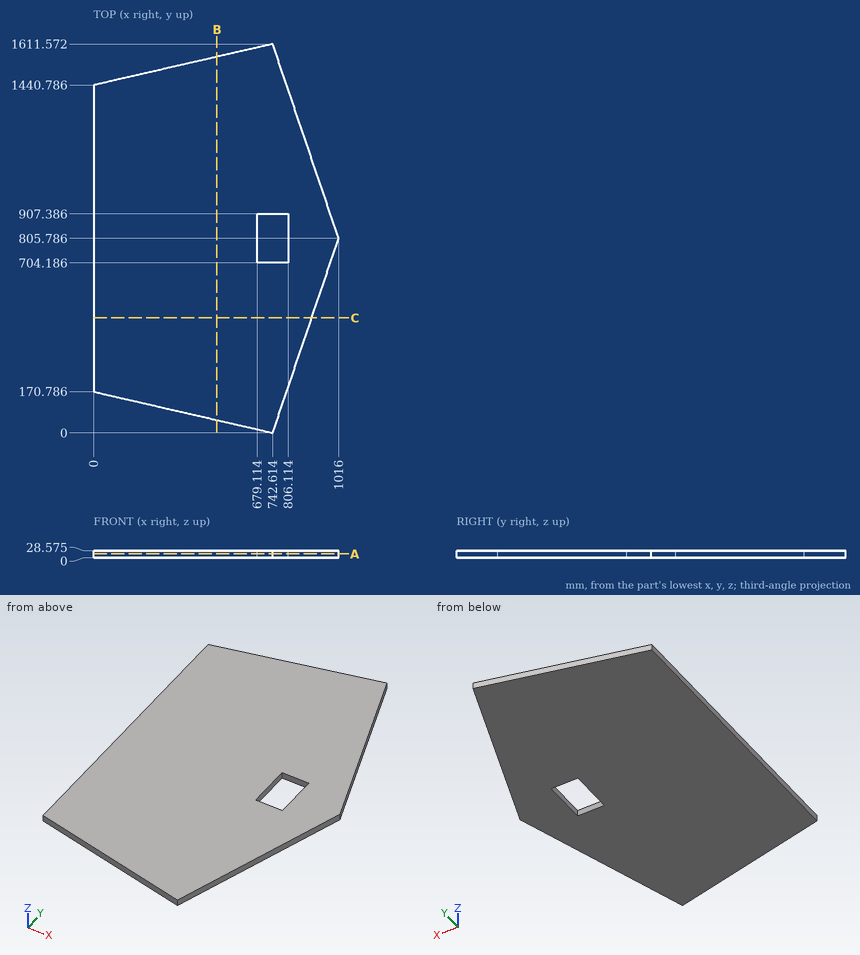
Could you check a few things on this drawing? It's one solid part, dimensions in mm from its lowest x, y, z. Coordinates: 2 decimals unless noted, no trailing zeros. Order: outer loops, then holes, each group sorted by start corner. A loop starts at its lowest first (then second) coordinate and runs counter-clockwise, first axis right, second up. Notation, with made-up numbers: M -25.75,15.25 L 22.25,15.25 A11 cw 22.25,36.25 Z; hole C -2.75,30 d4. An arc over 180 degrees is marked long. Use one line per item in the form item = value. Start each with the question number.
1. Suppose I cut it at B-B on x = 511.5. Write out the boundary of the cut face in (y, z) (1 decimal), then the cut area to 3 significant figures.
2. Suppose I cut it at C-C on y = 476.5. Write out the boundary of the cut face in (x, z) (1 decimal).
3. Suppose I cut it at A-A on z = 16.5. Write out the boundary of the cut face in (x, y) (1 decimal).
4. For pin 1 (1 mm diameter, centred on x = 492.5, z = 18.5, fed in from +Y); pin 2 (12 mm diameter, centred on x = 606, z = 16.5, fed in from -Y); pin 3 (4 mm diameter, centred on x = 250.5, z = 17.5, fed in from -Y), each with a flat end and sliding along its axis, tell me the tip position at first contact or that it passes through.
5. Please list where these lines run through material, in increasing order: line 1 (X direction, y = 1053, z = 10.5) (1 decimal); line 2 (Y direction, x = 721.5, z = 23.75) (1 decimal); line 3 (Y direction, x = 337, z = 3).
Geometry says:
q1.outline = M 53.2,0 L 1558.4,0 L 1558.4,28.6 L 53.2,28.6 Z
q1.area = 43,000 mm^2
q2.outline = M 0,0 L 904.3,0 L 904.3,28.6 L 0,28.6 Z
q3.outline = M 0,170.8 L 742.6,0 L 1016,805.8 L 742.6,1611.6 L 0,1440.8 Z; hole M 679.1,704.2 L 806.1,704.2 L 806.1,907.4 L 679.1,907.4 Z
q4.pin_1 = 1554.17
q4.pin_2 = 30.04
q4.pin_3 = 112.72
q5.line_1 = 0 to 932.1
q5.line_2 = 4.9 to 704.2, 907.4 to 1606.7
q5.line_3 = 93.28 to 1518.29
